```python
from build123d import *

# Parameters (mm, degrees)
F0_R     = 50.8
F1_DEPTH = 6.35
F2_R     = 19.05
F2_R_2   = 16.51
F3_DEPTH = 3.175


with BuildPart() as f1:
    # F0 (on Top) → F1 (new body)
    with BuildSketch(Plane.XY):
        Circle(F0_R)
    extrude(amount=F1_DEPTH)

    # F2 (on face) → F3 (cut)
    with BuildSketch(Plane.XY.offset(6.35)):
        with BuildLine():
            ThreePointArc((-27.064107, 14.965056), (-20.566075, 13.915697), (-18.50429, 7.664728))
            ThreePointArc((-18.50429, 7.664728), (-18.911897, 6.842578), (-19.419766, 6.078285))
            Line((-19.419766, 6.078285), (-23.875048, 6.888337))
            ThreePointArc((-23.875048, 6.888337), (-26.958737, 7.175685), (-29.128942, 4.96618))
            ThreePointArc((-29.128942, 4.96618), (-31.301297, 1.633058), (-35.279843, 1.634443))
            Line((-35.279843, 1.634443), (-42.498607, 5.606899))
            Line((-42.498607, 5.606899), (-36.826611, -2.354635))
            ThreePointArc((-36.826611, -2.354635), (-33.757711, -6.010738), (-29.719107, -8.555321))
            ThreePointArc((-29.719107, -8.555321), (-24.382295, -4.702528), (-18.50429, -7.664728))
            ThreePointArc((-18.50429, -7.664728), (-18.211164, -8.534298), (-18.029845, -9.433852))
            Line((-18.029845, -9.433852), (-21.752998, -12.011419))
            ThreePointArc((-21.752998, -12.011419), (-24.136681, -13.98873), (-24.108892, -17.085653))
            ThreePointArc((-24.108892, -17.085653), (-23.288106, -20.978613), (-26.102342, -23.79089))
            Line((-26.102342, -23.79089), (-34.01573, -26.086377))
            Line((-34.01573, -26.086377), (-24.375368, -27.705325))
            ThreePointArc((-24.375368, -27.705325), (-19.620073, -28.12054), (-14.965056, -27.064107))
            ThreePointArc((-14.965056, -27.064107), (-13.915697, -20.566075), (-7.664728, -18.50429))
            ThreePointArc((-7.664728, -18.50429), (-6.842578, -18.911897), (-6.078285, -19.419766))
            Line((-6.078285, -19.419766), (-6.888337, -23.875048))
            ThreePointArc((-6.888337, -23.875048), (-7.175685, -26.958737), (-4.96618, -29.128942))
            ThreePointArc((-4.96618, -29.128942), (-1.633058, -31.301297), (-1.634443, -35.279843))
            Line((-1.634443, -35.279843), (-5.606899, -42.498607))
            Line((-5.606899, -42.498607), (2.354635, -36.826611))
            ThreePointArc((2.354635, -36.826611), (6.010738, -33.757711), (8.555321, -29.719107))
            ThreePointArc((8.555321, -29.719107), (4.702528, -24.382295), (7.664728, -18.50429))
            ThreePointArc((7.664728, -18.50429), (8.534298, -18.211164), (9.433852, -18.029845))
            Line((9.433852, -18.029845), (12.011419, -21.752998))
            ThreePointArc((12.011419, -21.752998), (13.98873, -24.136681), (17.085653, -24.108892))
            ThreePointArc((17.085653, -24.108892), (20.978613, -23.288106), (23.79089, -26.102342))
            Line((23.79089, -26.102342), (26.086377, -34.01573))
            Line((26.086377, -34.01573), (27.705325, -24.375368))
            ThreePointArc((27.705325, -24.375368), (28.12054, -19.620073), (27.064107, -14.965056))
            ThreePointArc((27.064107, -14.965056), (20.566075, -13.915697), (18.50429, -7.664728))
            ThreePointArc((18.50429, -7.664728), (18.911897, -6.842578), (19.419766, -6.078285))
            Line((19.419766, -6.078285), (23.875048, -6.888337))
            ThreePointArc((23.875048, -6.888337), (26.958737, -7.175685), (29.128942, -4.96618))
            ThreePointArc((29.128942, -4.96618), (31.301297, -1.633058), (35.279843, -1.634443))
            Line((35.279843, -1.634443), (42.498607, -5.606899))
            Line((42.498607, -5.606899), (36.826611, 2.354635))
            ThreePointArc((36.826611, 2.354635), (33.757711, 6.010738), (29.719107, 8.555321))
            ThreePointArc((29.719107, 8.555321), (24.382295, 4.702528), (18.50429, 7.664728))
            ThreePointArc((18.50429, 7.664728), (18.211164, 8.534298), (18.029845, 9.433852))
            Line((18.029845, 9.433852), (21.752998, 12.011419))
            ThreePointArc((21.752998, 12.011419), (24.136681, 13.98873), (24.108892, 17.085653))
            ThreePointArc((24.108892, 17.085653), (23.288106, 20.978613), (26.102342, 23.79089))
            Line((26.102342, 23.79089), (34.01573, 26.086377))
            Line((34.01573, 26.086377), (24.375368, 27.705325))
            ThreePointArc((24.375368, 27.705325), (19.620073, 28.12054), (14.965056, 27.064107))
            ThreePointArc((14.965056, 27.064107), (13.915697, 20.566075), (7.664728, 18.50429))
            ThreePointArc((7.664728, 18.50429), (6.842578, 18.911897), (6.078285, 19.419766))
            Line((6.078285, 19.419766), (6.888337, 23.875048))
            ThreePointArc((6.888337, 23.875048), (7.175685, 26.958737), (4.96618, 29.128942))
            ThreePointArc((4.96618, 29.128942), (1.633058, 31.301297), (1.634443, 35.279843))
            Line((1.634443, 35.279843), (5.606899, 42.498607))
            Line((5.606899, 42.498607), (-2.354635, 36.826611))
            ThreePointArc((-2.354635, 36.826611), (-6.010738, 33.757711), (-8.555321, 29.719107))
            ThreePointArc((-8.555321, 29.719107), (-4.702528, 24.382295), (-7.664728, 18.50429))
            ThreePointArc((-7.664728, 18.50429), (-8.534298, 18.211164), (-9.433852, 18.029845))
            Line((-9.433852, 18.029845), (-12.011419, 21.752998))
            ThreePointArc((-12.011419, 21.752998), (-13.98873, 24.136681), (-17.085653, 24.108892))
            ThreePointArc((-17.085653, 24.108892), (-20.978613, 23.288106), (-23.79089, 26.102342))
            Line((-23.79089, 26.102342), (-26.086377, 34.01573))
            Line((-26.086377, 34.01573), (-27.705325, 24.375368))
            ThreePointArc((-27.705325, 24.375368), (-28.12054, 19.620073), (-27.064107, 14.965056))
        make_face()
        Circle(F2_R, mode=Mode.SUBTRACT)
        Circle(F2_R_2)
    extrude(amount=-F3_DEPTH, mode=Mode.SUBTRACT)


solid = f1.part
```
Model file for the job. Use its own axes, mm. Give positions to 0.01 mm unless a question says otherwise; leave off trailing zeros. Use a Markdown table: item, result.
1) Drill centre lines: line 1 (Y direction, x = 0, z = 4.1); line 2 (X direction, y = -20, z = 4.25); line 3 (X direction, y = -23, z = 5.25). Where is each one in solid material? Low to high. Write a range as from..to.
Responses:
| item | result |
|---|---|
| line 1 | y = -50.8..-38.5, -19.05..-16.51, 16.51..19.05, 38.5..50.8 |
| line 2 | x = -46.7..-23.12, -13.37..-6.18, 6.01..10.8, 28.14..46.7 |
| line 3 | x = -45.3..-24.62, -15.2..-6.73, 4.74..12.6, 27.98..45.3 |
2) Cut at A-A (z = 4.5). Give the number of separate pieces and of enclosed holes in the cut face, and give its area (3 significant figures).
Responses:
| item | result |
|---|---|
| separate pieces | 2 |
| enclosed holes | 2 |
| area | 5,610 mm2 |
3) Pull direction X, two halves, no side cores. Call faces 1 (the cylindrical face through (-13.98, -20.64, 4.78)), 2 (the cylindrical face through (-11.012, -49.592, 3.131)), 3 (the cylindrical face through (-23.27, -20.92, 4.78)): +X half, -X half, draft (parallel to the pull), parting line (faces both ways), or undercut.
Responses:
| item | result |
|---|---|
| face 1 | undercut |
| face 2 | parting line |
| face 3 | undercut |
4) Pin check, flat tips, straight feed: pin 1 (2 mm diameter, centred on y = -20.5, z = 5, fed in from +X); pin 2 (1 mm diameter, centred on x = 19, z = 4.5, fed in from -Y); pin 3 (10 mm diameter, centred on x = -3.5, y = 3.5, fed in from +Z) (3 decimals). Stop position of each tip, or through.
Responses:
| item | result |
|---|---|
| pin 1 | stops at x = 46.91 |
| pin 2 | stops at y = -47.31 |
| pin 3 | stops at z = 3.175 |
